from build123d import *

# Parameters (mm, degrees)
EXTRUDE_1_DEPTH        = 23.706666667
SKETCH_2_W             = 6.773333333
SKETCH_2_H             = 38.666666667
CUT_EXTRUDE_1_DEPTH    = 12.276666667
CHAMFER_1_SIZE         = 1
SKETCH_3_W             = 10.752666667
SKETCH_3_H             = 38.666666667
CUT_EXTRUDE_2_DEPTH    = 11.853333333
SKETCH_4_W             = 10.752666667
SKETCH_4_H             = 4.666666667
CUT_EXTRUDE_3_DEPTH    = 8.382
SKETCH_5_R             = 2.5
CUT_EXTRUDE_4_DEPTH    = 10
SKETCH_6_W             = 10.752666667
SKETCH_6_H             = 7.62
CUT_EXTRUDE_5_DEPTH    = 3
MIRROR_START           = 11.853333334
MIRROR_2_OUTLINE_W     = 10.752666667
MIRROR_2_OUTLINE_H     = 38.666666667
MIRROR_2_DEPTH         = 11.853333333
MIRROR_START_2         = 3.471333334
MIRROR_2_2_OUTLINE_W   = 10.752666667
MIRROR_2_2_OUTLINE_H   = 4.666666667
MIRROR_2_2_OUTLINE_H_2 = 4.666666668
MIRROR_2_2_OUTLINE_R   = 2.5
MIRROR_2_2_DEPTH       = 8.382
MIRROR_START_3         = 8.853333334
MIRROR_2_3_OUTLINE_W   = 10.752666667
MIRROR_2_3_OUTLINE_H   = 7.62
MIRROR_2_3_DEPTH       = 3
MIRROR_START_4         = 1.853333334
MIRROR_2_4_OUTLINE_R   = 2.5
MIRROR_2_4_DEPTH       = 1.618
MIRROR_START_5         = -19.333333333
MIRROR_2_5_DEPTH       = 38.666666667


# Read off the part's stored shape, not the designer's step: ﾐﾗｰ2
with BuildPart() as part:
    # ｽｹｯﾁ1 → ﾎﾞｽ - 押し出し1 (new body)
    with BuildSketch(Plane(origin=(0, 0, 0), x_dir=(1, 0, 0), z_dir=(0, 1, 0))):
        Polygon((-24.003333333, 19.333333333), (24.003333334, 19.333333333), (24.003333333, -19.333333334), (-24.003333333, -19.333333334), align=None)
    extrude(amount=EXTRUDE_1_DEPTH)

    # ｽｹｯﾁ2 → ｶｯﾄ - 押し出し1 (cut)
    with BuildSketch(Plane(origin=(0, 23.706666667, 0), x_dir=(1, 0, 0), z_dir=(0, 1, 0))):
        with Locations((20.616666667, -1e-09)):
            Rectangle(SKETCH_2_W, SKETCH_2_H)
    extrude(amount=-CUT_EXTRUDE_1_DEPTH, mode=Mode.SUBTRACT)

    # 面取り1
    chamfer_1_edges = [part.edges().sort_by_distance(p)[0] for p in [
        (24.003333334, 11.43, 0),
        (17.230000001, 23.706666667, 0),
    ]]
    chamfer(chamfer_1_edges, length=CHAMFER_1_SIZE)

    # ｽｹｯﾁ3 → ｶｯﾄ - 押し出し2 (cut)
    with BuildSketch(Plane(origin=(0, 23.706666667, 0), x_dir=(1, 0, 0), z_dir=(0, 1, 0))):
        with Locations((6.773666668, -1e-09)):
            Rectangle(SKETCH_3_W, SKETCH_3_H)
    extrude(amount=-CUT_EXTRUDE_2_DEPTH, mode=Mode.SUBTRACT)

    # ｽｹｯﾁ4 → ｶｯﾄ - 押し出し3 (cut)
    with BuildSketch(Plane(origin=(0, 11.853333334, 0), x_dir=(1, 0, 0), z_dir=(0, 1, 0))):
        with Locations((6.773666668, 17)):
            Rectangle(SKETCH_4_W, SKETCH_4_H)
    cut_extrude_3 = extrude(amount=-CUT_EXTRUDE_3_DEPTH, mode=Mode.SUBTRACT)

    # ｽｹｯﾁ5 → ｶｯﾄ - 押し出し4 (cut)
    with BuildSketch(Plane(origin=(0, 11.853333334, 0), x_dir=(1, 0, 0), z_dir=(0, 1, 0))):
        with Locations(Location((6.773666667, 9.593333333, 0), (0, 0, 270))):
            Circle(SKETCH_5_R)
    cut_extrude_4 = extrude(amount=-CUT_EXTRUDE_4_DEPTH, mode=Mode.SUBTRACT)

    # ﾐﾗｰ1: ｶｯﾄ - 押し出し3, ｶｯﾄ - 押し出し4 across plane
    add(cut_extrude_3.mirror(Plane.XY), mode=Mode.SUBTRACT)
    add(cut_extrude_4.mirror(Plane.XY), mode=Mode.SUBTRACT)

    # ｽｹｯﾁ6 → ｶｯﾄ - 押し出し5 (cut)
    with BuildSketch(Plane(origin=(0, 11.853333334, 0), x_dir=(1, 0, 0), z_dir=(0, 1, 0))):
        with Locations((6.773666668, 0.283333333)):
            Rectangle(SKETCH_6_W, SKETCH_6_H)
    extrude(amount=-CUT_EXTRUDE_5_DEPTH, mode=Mode.SUBTRACT)

    # ﾐﾗｰ2 outline → ﾐﾗｰ2 (cut)
    with BuildSketch(Plane(origin=(0, 0, 0), x_dir=(1, 0, 0), z_dir=(0, 1, 0)).offset(MIRROR_START)):
        with Locations((-6.773666668, -1e-09)):
            Rectangle(MIRROR_2_OUTLINE_W, MIRROR_2_OUTLINE_H)
    extrude(amount=MIRROR_2_DEPTH, mode=Mode.SUBTRACT)

    # Mirror 2 2 outline → Mirror 2 2 (cut)
    with BuildSketch(Plane(origin=(0, 0, 0), x_dir=(1, 0, 0), z_dir=(0, 1, 0)).offset(MIRROR_START_2)):
        with Locations((-6.773666668, 17)):
            Rectangle(MIRROR_2_2_OUTLINE_W, MIRROR_2_2_OUTLINE_H)
        with Locations((-6.773666668, -17)):
            Rectangle(MIRROR_2_2_OUTLINE_W, MIRROR_2_2_OUTLINE_H_2)
        with Locations((-6.773666667, 9.593333333)):
            Circle(MIRROR_2_2_OUTLINE_R)
        with Locations((-6.773666667, -9.593333333)):
            Circle(MIRROR_2_2_OUTLINE_R)
    extrude(amount=MIRROR_2_2_DEPTH, mode=Mode.SUBTRACT)

    # Mirror 2 3 outline → Mirror 2 3 (cut)
    with BuildSketch(Plane(origin=(0, 0, 0), x_dir=(1, 0, 0), z_dir=(0, 1, 0)).offset(MIRROR_START_3)):
        with Locations((-6.773666668, 0.283333333)):
            Rectangle(MIRROR_2_3_OUTLINE_W, MIRROR_2_3_OUTLINE_H)
    extrude(amount=MIRROR_2_3_DEPTH, mode=Mode.SUBTRACT)

    # Mirror 2 4 outline → Mirror 2 4 (cut)
    with BuildSketch(Plane(origin=(0, 0, 0), x_dir=(1, 0, 0), z_dir=(0, 1, 0)).offset(MIRROR_START_4)):
        with Locations((-6.773666667, 9.593333333)):
            Circle(MIRROR_2_4_OUTLINE_R)
        with Locations((-6.773666667, -9.593333333)):
            Circle(MIRROR_2_4_OUTLINE_R)
    extrude(amount=MIRROR_2_4_DEPTH, mode=Mode.SUBTRACT)

    # Mirror 2 5 outline → Mirror 2 5 (cut)
    with BuildSketch(Plane.XY.offset(MIRROR_START_5)):
        Polygon((-24.003333333, 23.706666667), (-24.003333333, 11.43), (-17.230000001, 11.43), (-17.230000001, 22.706666667), (-16.230000001, 23.706666667), align=None)
    extrude(amount=MIRROR_2_5_DEPTH, mode=Mode.SUBTRACT)


solid = part.part
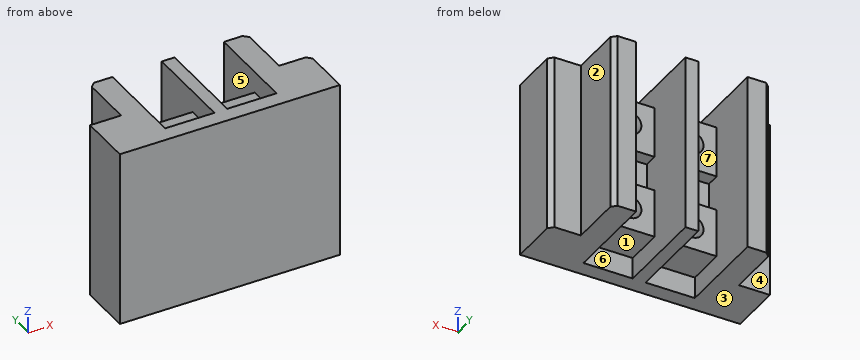
For this review, take the finished solid that the model builds, in its own axes (mm). Face numbers are marked on the shaded views. A direction names the side the tool comes from. Give positions to 0.01 mm unless a question says otherwise; leave off trailing zeros. Order: outer loops, then holes, each group sorted by start corner. A loop starts at its lowest first (then second) coordinate and runs counter-clockwise, first axis right, second up. Notation, with made-up numbers: (64, 5.25) -> (72, 5.25) arc R14 cw to (72, 30.25) -> close; hole circle Ø7 at (-9, 45.25). An arc over 180 degrees is marked (long way). Write item = value, one per line.
1) We need section D-D, the plane y = 8.25. Give the boundary of the cut face in (x, z), and give its area (3 significant figures).
Findings:
outline = (-24, -19.33) -> (-12.15, -19.33) -> (-12.15, -14.67) -> (-1.4, -14.67) -> (-1.4, -19.33) -> (1.4, -19.33) -> (1.4, -14.67) -> (12.15, -14.67) -> (12.15, -19.33) -> (24, -19.33) -> (24, 19.33) -> (12.15, 19.33) -> (12.15, 14.67) -> (1.4, 14.67) -> (1.4, 19.33) -> (-1.4, 19.33) -> (-1.4, 14.67) -> (-12.15, 14.67) -> (-12.15, 19.33) -> (-24, 19.33) -> close; hole circle Ø5 at (-6.77, -9.59); hole circle Ø5 at (-6.77, 9.59); hole circle Ø5 at (6.77, -9.59); hole circle Ø5 at (6.77, 9.59)
area = 1,580 mm^2
2) Insertion check: pin 1 (1.7 mm diameter, centred on x = 21.5, z = 6.5, fed in from +Y); pin 2 (4 mm diameter, centred on x = -5.5, y = 9, fed in from -Z); pin 3 (9 mm diameter, centred on y = 18.5, z = -9.5, fed in from -X). Each pin has a flat end and moves straight along its axis. Give the tip position at first contact, or say it passes through.
Findings:
pin_1 = 11.43
pin_2 = -14.67
pin_3 = -17.23
3) Draft analysis for pull direction X (two halves, no side actions). For the marked faces 1, 2 and 3, state which applies: pulls with the +X half, pulls with the -X half, needs draft (parallel to the pull), parting line crosses it, or undercut.
Findings:
face_1 = undercut
face_2 = pulls with the +X half
face_3 = needs draft
4) We need section A-A, the plane y = 15.25. Give the boundary of the cut face in (x, z).
Findings:
outline = (-17.23, -19.33) -> (-12.15, -19.33) -> (-12.15, 19.33) -> (-17.23, 19.33) -> close; (-1.4, -19.33) -> (1.4, -19.33) -> (1.4, 19.33) -> (-1.4, 19.33) -> close; (12.15, -19.33) -> (17.23, -19.33) -> (17.23, 19.33) -> (12.15, 19.33) -> close
5) We need section C-C, the plane z = -3. Give the boundary of the cut face in (x, y).
Findings:
outline = (-24, 0) -> (24, 0) -> (24, 10.43) -> (23, 11.43) -> (17.23, 11.43) -> (17.23, 22.71) -> (16.23, 23.71) -> (12.15, 23.71) -> (12.15, 8.85) -> (1.4, 8.85) -> (1.4, 23.71) -> (-1.4, 23.71) -> (-1.4, 8.85) -> (-12.15, 8.85) -> (-12.15, 23.71) -> (-16.23, 23.71) -> (-17.23, 22.71) -> (-17.23, 11.43) -> (-24, 11.43) -> close
6) We need section B-B, the plane x = -10.5. Give the boundary of the cut face in (y, z), and give its area (3 significant figures).
Findings:
outline = (0, -19.33) -> (3.47, -19.33) -> (3.47, -14.67) -> (11.85, -14.67) -> (11.85, -4.09) -> (8.85, -4.09) -> (8.85, 3.53) -> (11.85, 3.53) -> (11.85, 14.67) -> (3.47, 14.67) -> (3.47, 19.33) -> (0, 19.33) -> close
area = 357 mm^2
7) To check wall thickness, follow L1, parallel to X at y = 13.75, z = -9; L2, parallel to Z at x = -4, y = 10; L3, parallel to X at y = 7, z = 9.5. State the ranges of each line that lie inside material, in increasing order. Write a range as from..to.
Findings:
L1 = -17.23..-12.15, -1.4..1.4, 12.15..17.23
L2 = -14.67..-4.09, 3.53..14.67
L3 = -24..-9.27, -4.28..4.28, 9.27..24
8) For the marked faces 4, 5, 6 and 7, list the 3-axis set-ups (+Z, -Z, +X, -X, +Y, -Y) from which the entire face can be reached by the end or side of a thin tool; tool diameter is ignored.
Findings:
face_4 = +Z, -Z, -X, +Y
face_5 = +Y
face_6 = -Z, +Y
face_7 = +Z, -Z, +Y
